For this review, take the finished solid that the model builds, in its own axes (mm). Face numbers are marked on the shaded views. Round coordinates to 2 decimals unless told otherwise and drop trailing zeros. Write each loop counter-clockwise with the first axis right and the second up, starting at its lowest first coordinate (ties: lowest second). Pieces come first, ordered by that corner, then holes. Notation, with made-up numbers: (67, 62.25) -> (93, 62.25) arc R30 ccw to (93, 85.25) -> close; hole circle Ø8 at (-32, 17.5). An arc over 180 degrees is marked (long way). Answer in a Markdown table with one row per item.
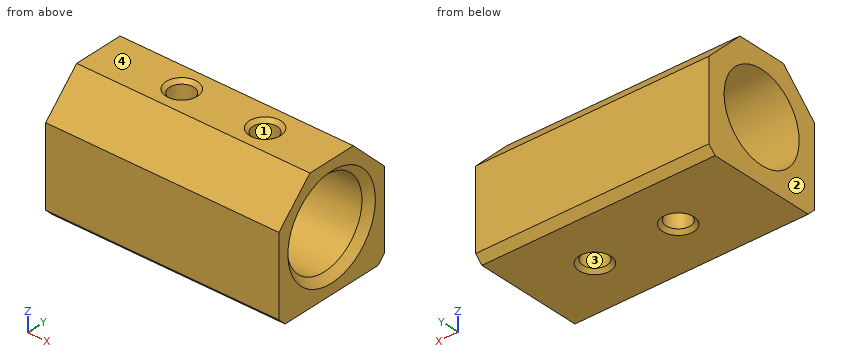
from build123d import *

# Parameters (mm, degrees)
SKETCH2_W           = 65
SKETCH2_H           = 34
BOSS_EXTRUDE1_DEPTH = 34
CHAMFER1_SIZE       = 10
CHAMFER2_SIZE       = 2
SKETCH3_R           = 12.1
CUT_EXTRUDE1_DEPTH  = 76.299402388
CHAMFER3_SIZE       = 2
SKETCH4_R           = 3.38
CUT_EXTRUDE2_DEPTH  = 51.012498438
CHAMFER4_SIZE       = 1


with BuildPart() as part:
    # Sketch2 → Boss-Extrude1 (new body)
    with BuildSketch(Plane.XY):
        Rectangle(SKETCH2_W, SKETCH2_H)
    extrude(amount=BOSS_EXTRUDE1_DEPTH)

    # Chamfer1
    chamfer1_edges = [part.edges().sort_by_distance(p)[0] for p in [
        (0, -17, 34),
        (0, 17, 34),
    ]]
    chamfer(chamfer1_edges, length=CHAMFER1_SIZE)

    # Chamfer2
    chamfer2_edges = [part.edges().sort_by_distance(p)[0] for p in [
        (0, -17, 0),
        (0, 17, 0),
    ]]
    chamfer(chamfer2_edges, length=CHAMFER2_SIZE)

    # Sketch3 → Cut-Extrude1 (cut, through all)
    with BuildSketch(Plane(origin=(32.5, 0, 0), x_dir=(0, 0, -1), z_dir=(1, 0, 0))):
        with Locations((-17, 0)):
            Circle(SKETCH3_R)
    extrude(amount=-CUT_EXTRUDE1_DEPTH, mode=Mode.SUBTRACT)

    # Chamfer3
    chamfer3_edges = [part.edges().sort_by_distance(p)[0] for p in [
        (32.5, 0, 29.1),
    ]]
    chamfer(chamfer3_edges, length=CHAMFER3_SIZE)

    # Sketch4 → Cut-Extrude2 (cut, through all)
    with BuildSketch(Plane.XY.offset(34)):
        with Locations((-9.27, 0)):
            Circle(SKETCH4_R)
        with Locations((13.96, 0)):
            Circle(SKETCH4_R)
    extrude(amount=-CUT_EXTRUDE2_DEPTH, mode=Mode.SUBTRACT)

    # Chamfer4
    chamfer4_edges = [part.edges().sort_by_distance(p)[0] for p in [
        (-12.65, 0, 0),
        (-12.65, 0, 34),
        (10.58, 0, 0),
        (10.58, 0, 34),
    ]]
    chamfer(chamfer4_edges, length=CHAMFER4_SIZE)


solid = part.part
1) For line 1 (X direction, y = 0, z = 31.95); line 2 (X direction, y = 0, z = 30.65); line 3 (Y direction, x = 4, z = 17), list the stretches that pass through material, from the lowest coordinate up. Write a range as [from, to].
Solved:
| item | result |
|---|---|
| line 1 | [-32.5, -12.65], [-5.89, 10.58], [17.34, 32.5] |
| line 2 | [-32.5, -12.65], [-5.89, 10.58], [17.34, 32.05] |
| line 3 | [-17, -12.1], [12.1, 17] |
2) Clearance check with flat-ended pins moving along their axes: pin 1 Ø6 at (y, z) = (0.5, 7.5) entering from +X; pin 2 Ø8 at (x, y) = (13.96, 0) entering from -Z; pin 3 Ø1.5 at (x, y) = (22, 9) entering from +Z; pin 4 Ø5.5 at (x, y) = (13.96, 0) entering from +Z. State where each tip first meets the part, or that it passes through.
Solved:
| item | result |
|---|---|
| pin 1 | x = 30.91 |
| pin 2 | z = 0.38 |
| pin 3 | z = 32.75 |
| pin 4 | through |
3) Consider section D-D on x = -4. State the section outline as (y, z) points, then the cut area to 3 significant figures.
Solved:
| item | result |
|---|---|
| outline | (-17, 2) -> (-15, 0) -> (15, 0) -> (17, 2) -> (17, 24) -> (7, 34) -> (-7, 34) -> (-17, 24) -> close; hole circle Ø24.2 at (0, 17) |
| area | 592 mm² |
4) Consider section B-B on x = 13.96. State the section outline as (y, z) points.
Solved:
| item | result |
|---|---|
| outline | (-17, 2) -> (-15, 0) -> (-4.38, 0) -> (-3.38, 1) -> (-3.38, 5.38) arc R12.1 cw to (-3.38, 28.62) -> (-3.38, 33) -> (-4.38, 34) -> (-7, 34) -> (-17, 24) -> close; (3.38, 1) -> (4.38, 0) -> (15, 0) -> (17, 2) -> (17, 24) -> (7, 34) -> (4.38, 34) -> (3.38, 33) -> (3.38, 28.62) arc R12.1 cw to (3.38, 5.38) -> close |
5) Consider section C-C on z = 17. State the section outline as (x, y) points, then the cut area to 3 significant figures.
Solved:
| item | result |
|---|---|
| outline | (-32.5, -17) -> (32.5, -17) -> (32.5, -14.1) -> (30.5, -12.1) -> (-32.5, -12.1) -> close; (-32.5, 12.1) -> (30.5, 12.1) -> (32.5, 14.1) -> (32.5, 17) -> (-32.5, 17) -> close |
| area | 633 mm² |
6) Consider section A-A on y = 0. State how many separate pieces and enclosed holes the cut face has, then the cut area to 3 significant figures.
Solved:
| item | result |
|---|---|
| separate pieces | 6 |
| enclosed holes | 0 |
| area | 497 mm² |
7) Mouldability with a two-part tool opening along X and no side actions: class the marked faces 1, 2, 3 and 4 as pulls with the +X half, pulls with the -X half, needs draft (parallel to the pull), parting line crosses it, or undercut.
Solved:
| item | result |
|---|---|
| face 1 | undercut |
| face 2 | pulls with the -X half |
| face 3 | undercut |
| face 4 | needs draft |
